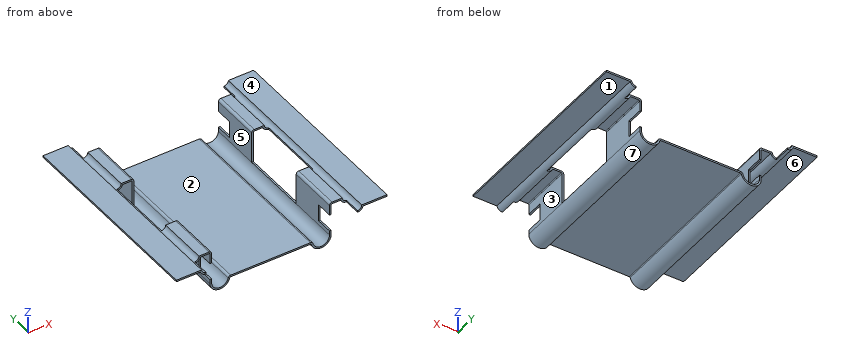
```python
from build123d import *

# Parameters (mm, degrees)
EXTRUDE_THIN1_DEPTH      = 6
EXTRUDE_THIN1_DEPTH_BACK = 6
SKETCH2_W                = 2
SKETCH2_H                = 4
SKETCH2_W_2              = 3
SKETCH2_H_2              = 1
EXTRUDE1_DEPTH           = 4.5
EXTRUDE1_DEPTH_BACK      = 4.5
SKETCH3_W                = 1
SKETCH3_H                = 1
EXTRUDE2_DEPTH           = 10
EXTRUDE2_DEPTH_BACK      = 10


with BuildPart() as part:
    # Sketch1 → Extrude-Thin1 (new body, two sides)
    with BuildSketch(Plane(origin=(0, 0, 0), x_dir=(1, 0, 0), z_dir=(0, 1, 0))) as extrude_thin1_sk:
        with BuildLine():
            Line((-6.25, 0), (-4.75, 0))
            ThreePointArc((-4.75, 0), (-4.5, 0.25), (-4.25, 0))
            Line((-4.25, 0), (-3.65, 0))
            ThreePointArc((-3.65, 0), (-3.543933983, 0.043933983), (-3.5, 0.15))
            Line((-3.5, 0.15), (-3.5, 2.001234471))
            ThreePointArc((-3.5, 2.001234471), (-3.058085593, 2.497849074), (-2.513495745, 2.116619086))
            ThreePointArc((-2.513495745, 2.116619086), (-2.460570519, 2.03356479), (-2.367544468, 2.001234471))
            Line((-2.367544468, 2.001234471), (2.367544468, 2.001234471))
            ThreePointArc((2.367544468, 2.001234471), (2.460570519, 2.03356479), (2.513495745, 2.116619086))
            ThreePointArc((2.513495745, 2.116619086), (3.058085593, 2.497849074), (3.5, 2.001234471))
            Line((3.5, 2.001234471), (3.5, 0.15))
            ThreePointArc((3.5, 0.15), (3.543933983, 0.043933983), (3.65, 0))
            Line((3.65, 0), (4.25, 0))
            ThreePointArc((4.25, 0), (4.5, 0.25), (4.75, 0))
            Line((4.75, 0), (6.25, 0))
            Line((6.25, 0), (6.25, 0.1))
            Line((6.25, 0.1), (4.835410197, 0.1))
            ThreePointArc((4.835410197, 0.1), (4.5, 0.35), (4.164589803, 0.1))
            Line((4.164589803, 0.1), (3.65, 0.1))
            ThreePointArc((3.65, 0.1), (3.614644661, 0.114644661), (3.6, 0.15))
            Line((3.6, 0.15), (3.6, 2.001234471))
            ThreePointArc((3.6, 2.001234471), (3.069702712, 2.597171994), (2.416194894, 2.139696009))
            ThreePointArc((2.416194894, 2.139696009), (2.398553152, 2.112011244), (2.367544468, 2.101234471))
            Line((2.367544468, 2.101234471), (-2.367544468, 2.101234471))
            ThreePointArc((-2.367544468, 2.101234471), (-2.398553152, 2.112011244), (-2.416194894, 2.139696009))
            ThreePointArc((-2.416194894, 2.139696009), (-3.069702712, 2.597171994), (-3.6, 2.001234471))
            Line((-3.6, 2.001234471), (-3.6, 0.15))
            ThreePointArc((-3.6, 0.15), (-3.614644661, 0.114644661), (-3.65, 0.1))
            Line((-3.65, 0.1), (-4.164589803, 0.1))
            ThreePointArc((-4.164589803, 0.1), (-4.5, 0.35), (-4.835410197, 0.1))
            Line((-4.835410197, 0.1), (-6.25, 0.1))
            Line((-6.25, 0.1), (-6.25, 0))
        make_face()
    extrude(amount=EXTRUDE_THIN1_DEPTH)
    extrude(extrude_thin1_sk.sketch, amount=-EXTRUDE_THIN1_DEPTH_BACK)

    # Sketch2 → Extrude1 (cut, two sides)
    with BuildSketch(Plane(origin=(0, 0, 0), x_dir=(0, 0, -1), z_dir=(1, 0, 0))) as extrude1_sk:
        with Locations((1, 0)):
            Rectangle(SKETCH2_W, SKETCH2_H)
        with Locations((1.5, -5.5)):
            Rectangle(SKETCH2_W_2, SKETCH2_H_2)
        with Locations((1.5, 5.5)):
            Rectangle(SKETCH2_W_2, SKETCH2_H_2)
    extrude(amount=EXTRUDE1_DEPTH, mode=Mode.SUBTRACT)
    extrude(extrude1_sk.sketch, amount=-EXTRUDE1_DEPTH_BACK, mode=Mode.SUBTRACT)

    # Sketch3 → Extrude2 (cut, two sides)
    with BuildSketch(Plane(origin=(0, 0, 0), x_dir=(0, 0, -1), z_dir=(1, 0, 0))) as extrude2_sk:
        with Locations((1.25, 4.5)):
            Rectangle(SKETCH3_W, SKETCH3_H)
        with Locations((1.25, -4.5)):
            Rectangle(SKETCH3_W, SKETCH3_H)
    extrude(amount=EXTRUDE2_DEPTH, mode=Mode.SUBTRACT)
    extrude(extrude2_sk.sketch, amount=-EXTRUDE2_DEPTH_BACK, mode=Mode.SUBTRACT)


solid = part.part
```
CAD build for the part. Positions are in the model's coordinates, mm. Face numbers are marked on the shaded views. A direction names the side the tool comes from. Round coordinates to 2 decimals unless told otherwise and drop trailing zeros. Write each loop counter-clockwise with the first axis right and the second up, starting at its lowest first coordinate (ties: lowest second). Pieces come first, ordered by that corner, then holes. Notation, with made-up numbers: (59, 86) - (82, 86) arc R18 cw to (82, 97) - close; hole circle Ø3 at (32, 35.25). An arc over 180 degrees is marked (long way). Return JSON: item names as keys, results as strings. Group by question number.
Item 1: Band-saw the part on D-D on x = 2. List the corners of the cut face in (y, z), plus the area to 3 significant figures.
Item 2: Band-saw the part on A-A on y = 1.75. State how many separate pieces and enclosed holes the cut face has, plus the area to 3 significant figures.
Item 3: Band-saw the part on B-B on z = -1.5. List the corners of the cut face in (x, y).
Item 4: 3-axis set-ups, long thin cutter, end or side, ignore diameter. For the marked faces 1, 2, 3 and 4: which of +Z, -Z, +X, -X, +Y, -Y reach the whole face in a straight line?
Item 5: Mould opens along X. For the marked faces 5, 6 and 7 say: +X half, -X half, draft (parallel to the pull), parting line (faces both ways), or undercut.
Item 6: Flat gauge pins, fed straight in: pin 1 Ø4 at (x, y) = (-1.5, -1) entering from -Z; pin 2 Ø1.1 at (x, z) = (4, -1) entering from -Y. Where does each tip first touch, or does it go through?
Resolved:
{
 "1": {"outline": "(-5, -2.1) - (5, -2.1) - (5, -2) - (-5, -2) - close", "area": "1.00 mm²"},
 "2": {"separate pieces": "3", "enclosed holes": "0", "area": "1.20 mm²"},
 "3": {"outline": "(-3.6, -4) - (-3.5, -4) - (-3.5, -2) - (-3.6, -2) - close; (-3.6, 2) - (-3.5, 2) - (-3.5, 4) - (-3.6, 4) - close; (3.5, -4) - (3.6, -4) - (3.6, -2) - (3.5, -2) - close; (3.5, 2) - (3.6, 2) - (3.6, 4) - (3.5, 4) - close"},
 "4": {"face 1": "-Z, +X, +Y, -Y", "face 2": "+Z, +Y, -Y", "face 3": "-Z, +Y, -Y", "face 4": "+Z, +X, -X, +Y, -Y"},
 "5": {"face 5": "undercut", "face 6": "draft", "face 7": "undercut"},
 "6": {"pin 1": "stops at z = -2.6", "pin 2": "stops at y = -5"}
}
